```python
from build123d import *

# Parameters (mm, degrees)
SKETCH1_R           = 10
BOSS_EXTRUDE1_DEPTH = 2
SKETCH2_R           = 4.5
BOSS_EXTRUDE2_DEPTH = 2.5
SKETCH3_R           = 1.275
CUT_EXTRUDE1_DEPTH  = 3
FILLET1_R           = 0.25
SKETCH6_R           = 1
CUT_EXTRUDE2_DEPTH  = 5.5
SKETCH7_R           = 2.9
CUT_EXTRUDE3_DEPTH  = 2.5
BOSS_EXTRUDE4_DEPTH = 2.5
CIRPATTERN1_COUNT   = 26


with BuildPart() as part:
    # Sketch1 → Boss-Extrude1 (new body)
    with BuildSketch(Plane(origin=(0, 0, 0), x_dir=(1, 0, 0), z_dir=(0, 1, 0))):
        Circle(SKETCH1_R)
    extrude(amount=BOSS_EXTRUDE1_DEPTH)

    # Sketch2 → Boss-Extrude2 (add)
    with BuildSketch(Plane(origin=(0, 0, 0), x_dir=(1, 0, 0), z_dir=(0, 1, 0))):
        Circle(SKETCH2_R)
    extrude(amount=-BOSS_EXTRUDE2_DEPTH)

    # Sketch3 → Cut-Extrude1 (cut, through all)
    with BuildSketch(Plane(origin=(0, 0, 0), x_dir=(1, 0, 0), z_dir=(0, 1, 0))):
        with Locations((0, 7)):
            Circle(SKETCH3_R)
        with Locations((-7, 0)):
            Circle(SKETCH3_R)
        with Locations((0, -7)):
            Circle(SKETCH3_R)
        with Locations((7, 0)):
            Circle(SKETCH3_R)
    extrude(amount=CUT_EXTRUDE1_DEPTH, mode=Mode.SUBTRACT)

    # Fillet1
    fillet1_edges = [part.edges().sort_by_distance(p)[0] for p in [
        (-10, 0, 0),
    ]]
    fillet(fillet1_edges, radius=FILLET1_R)

    # Sketch6 → Cut-Extrude2 (cut, through all)
    with BuildSketch(Plane(origin=(0, 2, 0), x_dir=(1, 0, 0), z_dir=(0, 1, 0))):
        Circle(SKETCH6_R)
    extrude(amount=-CUT_EXTRUDE2_DEPTH, mode=Mode.SUBTRACT)

    # Sketch7 → Cut-Extrude3 (cut)
    with BuildSketch(Plane.XZ.offset(2.5)):
        Circle(SKETCH7_R)
    extrude(amount=-CUT_EXTRUDE3_DEPTH, mode=Mode.SUBTRACT)

    # Sketch8 → Boss-Extrude4 (add)
    with BuildSketch(Plane.XZ.offset(2.5)):
        with BuildLine():
            Line((-2.35244742, -1.046531787), (-2.745588284, -0.933672842))
            ThreePointArc((-2.745588284, -0.933672842), (-2.649635472, -1.178741646), (-2.531859978, -1.414102207))
            Line((-2.531859978, -1.414102207), (-2.35244742, -1.046531787))
        make_face()
    boss_extrude4 = extrude(amount=-BOSS_EXTRUDE4_DEPTH)

    # CirPattern1: Boss-Extrude4 ×26 about axis
    cirpattern1_axis = Axis((0, 0, 0), (0, 1, 0))
    for i in range(1, CIRPATTERN1_COUNT):
        add(boss_extrude4.rotate(cirpattern1_axis, i * 360 / CIRPATTERN1_COUNT))


solid = part.part
```
Here's how the part is built. I have some questions about the finished solid (model axes, mm). A direction names the side the tool comes from. Give positions to 0.01 mm unless a question says otherwise; leave off trailing zeros. Answer as a JSON object with one key per item and string values. Group by question number.
Item 1: If we mould it in two halves opening along X, with no side actions, what happens to faces 3 (the flat face through (4.2, 0, 2)), 4 (the cylindrical face through (-2.17, 1.11, 9.76)), 5 (the cylindrical face through (-0.276, 0.986, -5.755))? For each: pulls with the +X half, pulls with the -X half, needs draft (parallel to the pull), parting line crosses it, or undercut.
Item 2: For P1, Ø6.5, axis at x = 1, z = -0.5, coming from the -Y side; P2, Ø4, axis at x = 0, z = -7, coming from the -Y side; P3, Ø1, axis at x = -6.5, y = -1, coming from the +Z side, each with a flat end and sliding along its axis, tell me the tip position at first contact or that it passes through.
Item 3: Please list where these lines run through material, in increasing order: probe 1 along X at (y, z) = (1.25, 0) (3 decimals); probe 2 along Y at (x, z) = (-3.5, -3.5).
Item 4: Which directions (+Z, -Z, +X, -X, +Y, -Y) give clear straight access to the entire face, cutting with the end or side of a thin tool? Please do faces 1 (the cylindrical face through (-0.59, -1.23, -4.46)), 2 (the cylindrical face through (5.726, 0.986, -0.056)).
Result set:
{
 "1": {"face 3": "needs draft", "face 4": "parting line crosses it", "face 5": "undercut"},
 "2": {"P1": "y = -2.5", "P2": "y = 0", "P3": "through"},
 "3": {"probe 1": "-10 to -8.275, -5.725 to -1, 1 to 5.725, 8.275 to 10", "probe 2": "0 to 2"},
 "4": {"face 1": "-Y", "face 2": "+Y, -Y"}
}
